from build123d import *

# Parameters (mm, degrees)
SKETCH1_R           = 3
BOSS_EXTRUDE1_DEPTH = 5


with BuildPart() as part:
    # Sketch1 → Boss-Extrude1 (new body)
    with BuildSketch(Plane(origin=(0, 0, 0), x_dir=(1, 0, 0), z_dir=(0, 1, 0))):
        Polygon((33.8816744, 72.09863232), (-10.595420339, 104.452736288), (-54.231730978, 70.973303889), (-29.88305287, 39.237805242), (-53.684676855, 20.976296661), (-78.033354964, 52.711795308), (-121.669665603, 19.232362909), (-103.331670223, -32.62048586), (-65.620507482, -19.283761946), (-55.617964547, -47.567134002), (-93.329127288, -60.903857915), (-74.991131907, -112.756706684), (-19.991131907, -112.756706684), (-19.991131907, -72.756706684), (10.008868093, -72.756706684), (10.008868093, -112.756706684), (65.008868093, -112.756706684), (79.784278091, -59.778529484), (40.969230286, -50.114572533), (48.214362749, -21.014674397), (87.843592635, -30.881341921), (102.619002633, 22.096835279), (58.141907894, 54.450939247), (34.611650463, 22.103961255), (10.351416969, 39.751654328), align=None)
        with Locations((-105.788667233, 25.573221778)):
            Circle(SKETCH1_R, mode=Mode.SUBTRACT)
        with Locations((-89.788667233, 25.573221778)):
            Circle(SKETCH1_R, mode=Mode.SUBTRACT)
        with Locations((-73.788667233, 25.573221778)):
            Circle(SKETCH1_R, mode=Mode.SUBTRACT)
        with Locations((-41.788667233, 25.573221778)):
            Circle(SKETCH1_R, mode=Mode.SUBTRACT)
        with Locations((-25.788667233, 25.573221778)):
            Circle(SKETCH1_R, mode=Mode.SUBTRACT)
        with Locations((-9.788667233, 25.573221778)):
            Circle(SKETCH1_R, mode=Mode.SUBTRACT)
        with Locations((6.211332767, 25.573221778)):
            Circle(SKETCH1_R, mode=Mode.SUBTRACT)
        with Locations((22.211332767, 25.573221778)):
            Circle(SKETCH1_R, mode=Mode.SUBTRACT)
        with Locations((54.211332767, 25.573221778)):
            Circle(SKETCH1_R, mode=Mode.SUBTRACT)
        with Locations((70.211332767, 25.573221778)):
            Circle(SKETCH1_R, mode=Mode.SUBTRACT)
        with Locations((86.211332767, 25.573221778)):
            Circle(SKETCH1_R, mode=Mode.SUBTRACT)
        with Locations((-106.074287638, 9.575771325)):
            Circle(SKETCH1_R, mode=Mode.SUBTRACT)
        with Locations((-90.074287638, 9.575771325)):
            Circle(SKETCH1_R, mode=Mode.SUBTRACT)
        with Locations((-74.074287638, 9.575771325)):
            Circle(SKETCH1_R, mode=Mode.SUBTRACT)
        with Locations((-58.074287638, 9.575771325)):
            Circle(SKETCH1_R, mode=Mode.SUBTRACT)
        with Locations((-42.074287638, 9.575771325)):
            Circle(SKETCH1_R, mode=Mode.SUBTRACT)
        with Locations((-26.074287638, 9.575771325)):
            Circle(SKETCH1_R, mode=Mode.SUBTRACT)
        with Locations((-10.074287638, 9.575771325)):
            Circle(SKETCH1_R, mode=Mode.SUBTRACT)
        with Locations((5.925712362, 9.575771325)):
            Circle(SKETCH1_R, mode=Mode.SUBTRACT)
        with Locations((21.925712362, 9.575771325)):
            Circle(SKETCH1_R, mode=Mode.SUBTRACT)
        with Locations((37.925712362, 9.575771325)):
            Circle(SKETCH1_R, mode=Mode.SUBTRACT)
        with Locations((53.925712362, 9.575771325)):
            Circle(SKETCH1_R, mode=Mode.SUBTRACT)
        with Locations((69.925712362, 9.575771325)):
            Circle(SKETCH1_R, mode=Mode.SUBTRACT)
        with Locations((85.925712362, 9.575771325)):
            Circle(SKETCH1_R, mode=Mode.SUBTRACT)
        with Locations((-90.359908044, -6.421679127)):
            Circle(SKETCH1_R, mode=Mode.SUBTRACT)
        with Locations((-74.359908044, -6.421679127)):
            Circle(SKETCH1_R, mode=Mode.SUBTRACT)
        with Locations((-58.359908044, -6.421679127)):
            Circle(SKETCH1_R, mode=Mode.SUBTRACT)
        with Locations((-42.359908044, -6.421679127)):
            Circle(SKETCH1_R, mode=Mode.SUBTRACT)
        with Locations((-26.359908044, -6.421679127)):
            Circle(SKETCH1_R, mode=Mode.SUBTRACT)
        with Locations((-10.359908044, -6.421679127)):
            Circle(SKETCH1_R, mode=Mode.SUBTRACT)
        with Locations((5.640091956, -6.421679127)):
            Circle(SKETCH1_R, mode=Mode.SUBTRACT)
        with Locations((21.640091956, -6.421679127)):
            Circle(SKETCH1_R, mode=Mode.SUBTRACT)
        with Locations((37.640091956, -6.421679127)):
            Circle(SKETCH1_R, mode=Mode.SUBTRACT)
        with Locations((53.640091956, -6.421679127)):
            Circle(SKETCH1_R, mode=Mode.SUBTRACT)
        with Locations((69.640091956, -6.421679127)):
            Circle(SKETCH1_R, mode=Mode.SUBTRACT)
        with Locations((85.640091956, -6.421679127)):
            Circle(SKETCH1_R, mode=Mode.SUBTRACT)
        with Locations((-58.645528449, -22.41912958)):
            Circle(SKETCH1_R, mode=Mode.SUBTRACT)
        with Locations((-42.645528449, -22.41912958)):
            Circle(SKETCH1_R, mode=Mode.SUBTRACT)
        with Locations((-26.645528449, -22.41912958)):
            Circle(SKETCH1_R, mode=Mode.SUBTRACT)
        with Locations((-10.645528449, -22.41912958)):
            Circle(SKETCH1_R, mode=Mode.SUBTRACT)
        with Locations((5.354471551, -22.41912958)):
            Circle(SKETCH1_R, mode=Mode.SUBTRACT)
        with Locations((21.354471551, -22.41912958)):
            Circle(SKETCH1_R, mode=Mode.SUBTRACT)
        with Locations((37.354471551, -22.41912958)):
            Circle(SKETCH1_R, mode=Mode.SUBTRACT)
        with Locations((69.354471551, -22.41912958)):
            Circle(SKETCH1_R, mode=Mode.SUBTRACT)
        with Locations((-42.931148854, -38.416580032)):
            Circle(SKETCH1_R, mode=Mode.SUBTRACT)
        with Locations((-26.931148854, -38.416580032)):
            Circle(SKETCH1_R, mode=Mode.SUBTRACT)
        with Locations((-10.931148854, -38.416580032)):
            Circle(SKETCH1_R, mode=Mode.SUBTRACT)
        with Locations((5.068851146, -38.416580032)):
            Circle(SKETCH1_R, mode=Mode.SUBTRACT)
        with Locations((21.068851146, -38.416580032)):
            Circle(SKETCH1_R, mode=Mode.SUBTRACT)
        with Locations((37.068851146, -38.416580032)):
            Circle(SKETCH1_R, mode=Mode.SUBTRACT)
        with Locations((-59.216769259, -54.414030485)):
            Circle(SKETCH1_R, mode=Mode.SUBTRACT)
        with Locations((-43.216769259, -54.414030485)):
            Circle(SKETCH1_R, mode=Mode.SUBTRACT)
        with Locations((-27.216769259, -54.414030485)):
            Circle(SKETCH1_R, mode=Mode.SUBTRACT)
        with Locations((-11.216769259, -54.414030485)):
            Circle(SKETCH1_R, mode=Mode.SUBTRACT)
        with Locations((4.783230741, -54.414030485)):
            Circle(SKETCH1_R, mode=Mode.SUBTRACT)
        with Locations((20.783230741, -54.414030485)):
            Circle(SKETCH1_R, mode=Mode.SUBTRACT)
        with Locations((36.783230741, -54.414030485)):
            Circle(SKETCH1_R, mode=Mode.SUBTRACT)
        with Locations((-75.502389665, -70.411480938)):
            Circle(SKETCH1_R, mode=Mode.SUBTRACT)
        with Locations((-59.502389665, -70.411480938)):
            Circle(SKETCH1_R, mode=Mode.SUBTRACT)
        with Locations((-43.502389665, -70.411480938)):
            Circle(SKETCH1_R, mode=Mode.SUBTRACT)
        with Locations((-27.502389665, -70.411480938)):
            Circle(SKETCH1_R, mode=Mode.SUBTRACT)
        with Locations((20.497610335, -70.411480938)):
            Circle(SKETCH1_R, mode=Mode.SUBTRACT)
        with Locations((36.497610335, -70.411480938)):
            Circle(SKETCH1_R, mode=Mode.SUBTRACT)
        with Locations((52.497610335, -70.411480938)):
            Circle(SKETCH1_R, mode=Mode.SUBTRACT)
        with Locations((68.497610335, -70.411480938)):
            Circle(SKETCH1_R, mode=Mode.SUBTRACT)
        with Locations((-75.78801007, -86.40893139)):
            Circle(SKETCH1_R, mode=Mode.SUBTRACT)
        with Locations((-59.78801007, -86.40893139)):
            Circle(SKETCH1_R, mode=Mode.SUBTRACT)
        with Locations((-43.78801007, -86.40893139)):
            Circle(SKETCH1_R, mode=Mode.SUBTRACT)
        with Locations((-27.78801007, -86.40893139)):
            Circle(SKETCH1_R, mode=Mode.SUBTRACT)
        with Locations((20.21198993, -86.40893139)):
            Circle(SKETCH1_R, mode=Mode.SUBTRACT)
        with Locations((36.21198993, -86.40893139)):
            Circle(SKETCH1_R, mode=Mode.SUBTRACT)
        with Locations((52.21198993, -86.40893139)):
            Circle(SKETCH1_R, mode=Mode.SUBTRACT)
        with Locations((68.21198993, -86.40893139)):
            Circle(SKETCH1_R, mode=Mode.SUBTRACT)
        with Locations((-60.073630475, -102.406381843)):
            Circle(SKETCH1_R, mode=Mode.SUBTRACT)
        with Locations((-44.073630475, -102.406381843)):
            Circle(SKETCH1_R, mode=Mode.SUBTRACT)
        with Locations((-28.073630475, -102.406381843)):
            Circle(SKETCH1_R, mode=Mode.SUBTRACT)
        with Locations((19.926369525, -102.406381843)):
            Circle(SKETCH1_R, mode=Mode.SUBTRACT)
        with Locations((35.926369525, -102.406381843)):
            Circle(SKETCH1_R, mode=Mode.SUBTRACT)
        with Locations((51.926369525, -102.406381843)):
            Circle(SKETCH1_R, mode=Mode.SUBTRACT)
        with Locations((-25.217426422, 57.568122683)):
            Circle(SKETCH1_R, mode=Mode.SUBTRACT)
        with Locations((-9.217426422, 57.568122683)):
            Circle(SKETCH1_R, mode=Mode.SUBTRACT)
        with Locations((6.782573578, 57.568122683)):
            Circle(SKETCH1_R, mode=Mode.SUBTRACT)
        with Locations((-24.931806017, 73.565573136)):
            Circle(SKETCH1_R, mode=Mode.SUBTRACT)
        with Locations((-8.931806017, 73.565573136)):
            Circle(SKETCH1_R, mode=Mode.SUBTRACT)
        with Locations((7.068193983, 73.565573136)):
            Circle(SKETCH1_R, mode=Mode.SUBTRACT)
        with Locations((23.068193983, 73.565573136)):
            Circle(SKETCH1_R, mode=Mode.SUBTRACT)
        with Locations((-8.646185612, 89.563023589)):
            Circle(SKETCH1_R, mode=Mode.SUBTRACT)
        with Locations((54.496953172, 41.570672231)):
            Circle(SKETCH1_R, mode=Mode.SUBTRACT)
        with Locations((6.496953172, 41.570672231)):
            Circle(SKETCH1_R, mode=Mode.SUBTRACT)
        with Locations((-9.503046828, 41.570672231)):
            Circle(SKETCH1_R, mode=Mode.SUBTRACT)
        with Locations((-25.503046828, 41.570672231)):
            Circle(SKETCH1_R, mode=Mode.SUBTRACT)
    extrude(amount=BOSS_EXTRUDE1_DEPTH)


solid = part.part
Design review of the part built by this model. Coordinates are the model's own, in mm. Round coordinates to 2 decimals unless told otherwise and drop trailing zeros. Order: outer loops, then holes, each group sorted by start corner. A loop starts at its lowest first (then second) coordinate and runs counter-clockwise, first axis right, second up. Notation, with made-up numbers: M 8,-40 L 24,-40 A15 cw 24,-36 Z; hole C 9,7 d7. An arc over 180 degrees is marked long. Answer as CSV lines item,"result". Start each with the question number.
1) Wall thickness on line 1 along X through (y, z) = (3.6, 79.5); line 2 along X through (y, z) = (1.8, 94.5); line 3 along Z through (x, y) = (48.5, 0.3): over which ranges is each line inside the solid? List them lowest first. Write a range as [from, to].
2) Add section B-B (z = 96.5). Give the boundary of the cut face in (x, y), then the cut area to 3 significant figures.
3) The part is to be moulded in two halves that separate along Z. For faces 1 (the face through (22.651, 2.465, -30.804)), 2 (the face through (19.214, 2.465, -25.705)), 3 (the face through (95.13, 2.46, 4.76)), say which applies: +Z half, -Z half, draft (parallel to the pull), parting line (faces both ways), or undercut.
4) Add section C-C (y = 3.25). Give the number of separate pieces and of enclosed holes in the cut face, then the cut area to 3 significant figures.
5) Add section A-A (z = -31.5). Give the boundary of the cut face in (x, y).
6) For pin 1 Ø1 at (y, z) = (1.5, 67) entering from +X; pin 2 Ø2 at (y, z) = (4, 7.5) entering from +X; pin 3 Ø1 at (y, z) = (2, 61) entering from -X, all flat-tipped, find the tip position at first contact; note any pin that passes through.
Resolved:
1,line 1,"[-86.75, -19.99], [10.01, 74.28]"
1,line 2,"[-81.45, -19.99], [10.01, 70.1]"
1,line 3,"[-41.2, 21.09], [51.99, 112.76]"
2,outline,"M -80.74,0 L -19.99,0 L -19.99,5 L -80.74,5 Z; M 10.01,0 L 69.54,0 L 69.54,5 L 10.01,5 Z"
2,area,"601 mm^2"
3,face 1,"undercut"
3,face 2,"undercut"
3,face 3,"+Z half"
4,separate pieces,"1"
4,enclosed holes,"91"
4,area,"25,100 mm^2"
5,outline,"M -105.68,0 L -61.76,0 L -61.76,5 L -105.68,5 Z; M -39.97,0 L 21.69,0 L 21.69,5 L -39.97,5 Z; M 41.45,0 L 89.69,0 L 89.69,5 L 41.45,5 Z"
6,pin 1,"x = 77.91"
6,pin 2,"x = 94.64"
6,pin 3,"x = -93.33"
